The listing builds one solid part. Answer for the finished solid, in the listing's coordinates (mm). Face numbers are marked on the shaded views. Round coordinates to 2 decimals unless told otherwise and drop trailing zeros. Loops run counter-clockwise (first coordinate to the right, second up) from the corner with the lowest first, then second, coordinate; pieces in that order, holes last. Notation, with made-up numbers: (83.25, 58.25) - (102.25, 58.25) arc R23 cw to (102.25, 89.25) - close; hole circle Ø5 at (-36.75, 35.25). An arc over 180 degrees is marked (long way). One line per item, written item: value.
```python
from build123d import *

# Parameters (mm, degrees)
SKETCH1_R           = 3
BOSS_EXTRUDE1_DEPTH = 3
CUT_EXTRUDE1_START  = 1.5
CUT_EXTRUDE1_DEPTH  = 6
CUT_EXTRUDE2_START  = -7.5
CUT_EXTRUDE2_DEPTH  = 6
CHAMFER1_SIZE       = 0.5


with BuildPart() as part:
    # Sketch1 → Boss-Extrude1 (new, symmetric)
    with BuildSketch(Plane(origin=(0, 0, 0), x_dir=(1, 0, 0), z_dir=(0, 1, 0))):
        with BuildLine():
            Line((-31, 6), (31, 6))
            ThreePointArc((31, 6), (37, 0), (31, -6))
            Line((31, -6), (-31, -6))
            ThreePointArc((-31, -6), (-37, 0), (-31, 6))
        make_face()
        with Locations(Location((-31, 0, 0), (0, 0, 270))):
            Circle(SKETCH1_R, mode=Mode.SUBTRACT)
        with Locations(Location((31, 0, 0), (0, 0, 90))):
            Circle(SKETCH1_R, mode=Mode.SUBTRACT)
        with Locations(Location((0, 0, 0), (0, 0, 270))):
            Circle(SKETCH1_R, mode=Mode.SUBTRACT)
        with Locations(Location((10, 0, 0), (0, 0, 270))):
            Circle(SKETCH1_R, mode=Mode.SUBTRACT)
        with Locations(Location((20, 0, 0), (0, 0, 270))):
            Circle(SKETCH1_R, mode=Mode.SUBTRACT)
        with Locations(Location((-20, 0, 0), (0, 0, 90))):
            Circle(SKETCH1_R, mode=Mode.SUBTRACT)
        with Locations(Location((-10, 0, 0), (0, 0, 90))):
            Circle(SKETCH1_R, mode=Mode.SUBTRACT)
    extrude(amount=BOSS_EXTRUDE1_DEPTH, both=True)

    # Sketch2 → Cut-Extrude1 (cut)
    with BuildSketch(Plane(origin=(0, 0, 0), x_dir=(1, 0, 0), z_dir=(0, 1, 0)).offset(CUT_EXTRUDE1_START)):
        with BuildLine():
            Line((-26.641101056, 4.75), (26.641101056, 4.75))
            ThreePointArc((26.641101056, 4.75), (27.549994316, 4.167028828), (27.399170438, 3.097826087))
            ThreePointArc((27.399170438, 3.097826087), (26.25, 0), (27.399170438, -3.097826087))
            ThreePointArc((27.399170438, -3.097826087), (27.549994316, -4.167028828), (26.641101056, -4.75))
            Line((26.641101056, -4.75), (-26.641101056, -4.75))
            ThreePointArc((-26.641101056, -4.75), (-27.549994316, -4.167028828), (-27.399170438, -3.097826087))
            ThreePointArc((-27.399170438, -3.097826087), (-26.25, 0), (-27.399170438, 3.097826087))
            ThreePointArc((-27.399170438, 3.097826087), (-27.549994316, 4.167028828), (-26.641101056, 4.75))
        make_face()
    extrude(amount=CUT_EXTRUDE1_DEPTH, mode=Mode.SUBTRACT)

    # Sketch2_2 → Cut-Extrude2 (cut)
    with BuildSketch(Plane(origin=(0, 0, 0), x_dir=(1, 0, 0), z_dir=(0, 1, 0)).offset(CUT_EXTRUDE2_START)):
        with BuildLine():
            Line((-26.641101056, 4.75), (26.641101056, 4.75))
            ThreePointArc((26.641101056, 4.75), (27.549994316, 4.167028828), (27.399170438, 3.097826087))
            ThreePointArc((27.399170438, 3.097826087), (26.25, 0), (27.399170438, -3.097826087))
            ThreePointArc((27.399170438, -3.097826087), (27.549994316, -4.167028828), (26.641101056, -4.75))
            Line((26.641101056, -4.75), (-26.641101056, -4.75))
            ThreePointArc((-26.641101056, -4.75), (-27.549994316, -4.167028828), (-27.399170438, -3.097826087))
            ThreePointArc((-27.399170438, -3.097826087), (-26.25, 0), (-27.399170438, 3.097826087))
            ThreePointArc((-27.399170438, 3.097826087), (-27.549994316, 4.167028828), (-26.641101056, 4.75))
        make_face()
    extrude(amount=CUT_EXTRUDE2_DEPTH, mode=Mode.SUBTRACT)

    # Chamfer1
    chamfer1_edges = [part.edges().sort_by_distance(p)[0] for p in [
        (-31, -3, -3),
        (-31, 3, -3),
        (37, 3, 0),
        (31, -3, 3),
        (31, 3, 3),
        (0, 3, -6),
        (0, 3, -4.75),
        (27.549994316, 3, -4.167028828),
        (26.25, 3, 0),
        (27.549994316, 3, 4.167028828),
        (0, 3, 4.75),
        (-27.549994316, 3, 4.167028828),
        (-26.25, 3, 0),
        (-27.549994316, 3, -4.167028828),
        (-27.549994316, 1.5, -4.167028828),
        (-37, 3, 0),
        (0, -3, -6),
        (-26.25, 1.5, 0),
        (-27.549994316, 1.5, 4.167028828),
        (0, 1.5, 4.75),
        (27.549994316, 1.5, 4.167028828),
        (26.25, 1.5, 0),
        (27.549994316, 1.5, -4.167028828),
        (0, 1.5, -4.75),
        (37, -3, 0),
        (0, 1.5, -3),
        (10, 1.5, -3),
        (20, 1.5, -3),
        (-20, 1.5, 3),
        (-10, 1.5, 3),
        (0, -3, 6),
        (-37, -3, 0),
        (-26.25, -3, 0),
        (-27.549994316, -3, 4.167028828),
        (0, -3, 4.75),
        (27.549994316, -3, 4.167028828),
        (26.25, -3, 0),
        (27.549994316, -3, -4.167028828),
        (0, -3, -4.75),
        (-27.549994316, -3, -4.167028828),
        (0, -1.5, -3),
        (10, -1.5, -3),
        (20, -1.5, -3),
        (0, 3, 6),
        (-20, -1.5, 3),
        (-10, -1.5, 3),
        (-27.549994316, -1.5, -4.167028828),
        (-26.25, -1.5, 0),
        (-27.549994316, -1.5, 4.167028828),
        (0, -1.5, 4.75),
        (27.549994316, -1.5, 4.167028828),
        (26.25, -1.5, 0),
        (27.549994316, -1.5, -4.167028828),
        (0, -1.5, -4.75),
    ]]
    chamfer(chamfer1_edges, length=CHAMFER1_SIZE)


solid = part.part
```
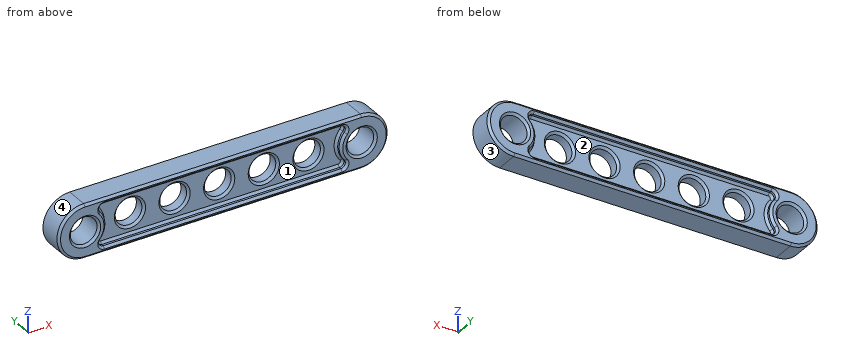
1) For a pull along X with two mould halves and no side action, classify the marked faces 1, 2, 3 and 4 as released by +X, released by -X, zero draft, split by the parting line, or undercut.
Final values:
face 1: undercut
face 2: undercut
face 3: released by +X
face 4: released by -X
2) Consider L1, parallel to Z at x = 31, y = 1; L2, parallel to X at y = 2.25, z = 2.75; L3, parallel to Z at x = 22.5, y = -2.25. Determine where each line is inside the solid, lowest interval first.
Final values:
L1: -6 to -3, 3 to 6
L2: -36.33 to -32.2, -29.8 to -27.13, 27.13 to 29.8, 32.2 to 36.33
L3: -6 to -4.75, 4.75 to 6
3) A cutting plane is placed at C-C on z = 1.5. Give the number of separate pieces and of enclosed holes in the cut face, and give its area (3 significant figures).
Final values:
separate pieces: 8
enclosed holes: 0
area: 138 mm2
4) Each of these flat-tipped pins is pushed along its axis until it touches: pin 1 Ø5 at (x, z) = (-31, 0) entering from -Y; pin 2 Ø7 at (x, z) = (4.5, 1) entering from -Y; pin 3 Ø7 at (x, z) = (-4.5, -0.5) entering from +Y. Where does it stop, or does it pass through?
Final values:
pin 1: through
pin 2: y = -1.75
pin 3: y = 1.5
5) A cutting plane is placed at B-B on y = 0. Give the vertices of the cut face in (x, z), and give its area (3 significant figures).
Final values:
outline: (-31, -6) - (31, -6) arc R6 ccw to (31, 6) - (-31, 6) arc R6 ccw to start; hole circle Ø6 at (-31, 0); hole circle Ø6 at (-20, 0); hole circle Ø6 at (-10, 0); hole circle Ø6 at (0, 0); hole circle Ø6 at (10, 0); hole circle Ø6 at (20, 0); hole circle Ø6 at (31, 0)
area: 659 mm2
